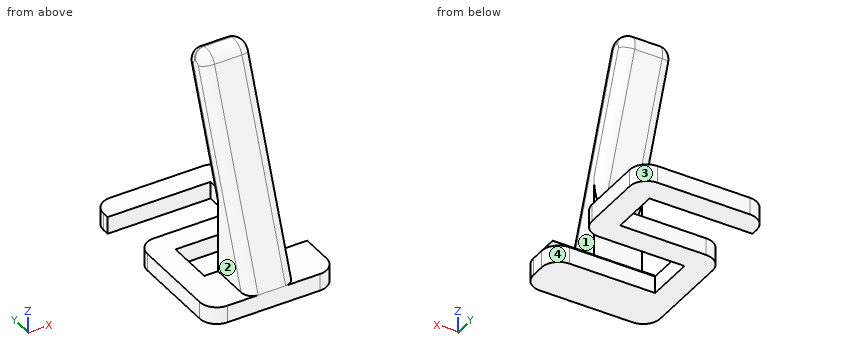
from build123d import *

# Parameters (mm, degrees)
F1_DEPTH = 5
F3_DEPTH = 37
F5_DEPTH = 36.2749
F6_R     = 4
F7_R     = 3
F8_R     = 4.99999


# Not quite as in the source:
# - a fillet or chamfer is up to 0.001 mm smaller than in the source, because OpenCascade refuses the exact size


with BuildPart() as f1:
    # F0 (on Top) → F1 (new body)
    with BuildSketch(Plane.XY):
        Polygon((0, 35), (0, 0), (37, 0), (37, 14), (7, 14), (7, 28), (37, 28), (37, 35), (37, 56), (0, 56), (0, 49), (30, 49), (30, 35), align=None)
    extrude(amount=F1_DEPTH)

    # F2 (on Right) → F3 (join)
    with BuildSketch(Plane.YZ):
        Polygon((22.2313093162, 66.0800203511), (0, 5), (9, 5), (14.2503125495, 4.9267373979), (14.2503125495, 19.4251151749), (30.1785093102, 63.1874761075), align=None)
    extrude(amount=F3_DEPTH)

    # F4 (on Front) → F5 (cut)
    with BuildSketch(Plane.XZ):
        Polygon((11, 5), (11, 66.0800203511), (25, 66.0800203511), (25, 5), (61.9937415394, 5), (61.9937415394, 77.6014764043), (-15.3317964795, 77.6014764043), (-15.3317964795, 5), align=None)
    extrude(amount=-F5_DEPTH, mode=Mode.SUBTRACT)

    # F6
    f6_edges = [f1.edges().sort_by_distance(p)[0] for p in [
        (18, 22.231309, 66.08002),
        (18, 30.178509, 63.187476),
    ]]
    fillet(f6_edges, radius=F6_R)

    # F7
    f7_edges = [f1.edges().sort_by_distance(p)[0] for p in [
        (11, 21.530371, 39.42691),
        (11, 10.431614, 33.660625),
        (25, 21.530371, 39.42691),
        (25, 10.431614, 33.660625),
    ]]
    fillet(f7_edges, radius=F7_R)

    # F8 (radius 5 in the source; OpenCascade refuses exactly that, so slightly less here)
    f8_edges = [f1.edges().sort_by_distance(p)[0] for p in [
        (37, 0, 2.5),
        (37, 28, 2.5),
        (37, 14, 2.465115),
        (0, 0, 2.5),
        (0, 35, 2.5),
        (0, 56, 2.5),
        (37, 56, 2.5),
    ]]
    fillet(f8_edges, radius=F8_R)


solid = f1.part
Design review of the part built by this model. Coordinates are the model's own, in mm. Face numbers are marked on the shaded views. A direction names the side the tool comes from. Coordinates: 2 decimals unless noted, no trailing zeros. Loops run counter-clockwise (first coordinate to the right, second up) from the corner with the lowest first, then second, coordinate; pieces in that order, holes last. Notation, with made-up numbers: (88.25, 15) -> (113.25, 15) arc R14 cw to (113.25, 40) -> close; hole circle Ø9 at (-9.5, 46.25). An arc over 180 degrees is marked (long way). Use a Markdown table: item, result. Add a question column.
Item 1: Wall thickness on L1, parallel to Z at x = 19.5, y = 53; L2, parallel to X at y = 13.5, z = 27; L3, parallel to Y at x = 12, z = 44.5: over which ranges is each line inside the solid? List them lowest first. Write a range as from..to.
Item 2: We need section C-C, the plane y = 42. Write out the cut boundary in (x, z), and give its area (3 significant figures).
Item 3: Machinability: for the marked faces 1, 2, 3 and 4, which of the approach directions +Z, -Z, +X, -X, +Y, -Y give a long, thin tool a straight path to every point of the face, cutting with its end or side? Answer none if there is none.
Item 4: Clearance check with flat-ended pins moving along their axes: P1, Ø1.5, axis at y = 22.5, z = 1.5, coming from the +X side; P2, Ø12, axis at x = 5.5, y = 47.5, coming from the +Z side; P3, Ø8, axis at x = 17.5, z = 38, coming from the -Y side; P4, Ø18.5, axis at x = 21.5, y = 31.5, coming from the +Z side. State where each tip first meets the part, or that it passes through.
Item 5: We need section A-A, the plane x = 10. Write out the cut boundary in (y, z).
Item 6: We need section B-B, the plane x = 18. Write out the cut boundary in (y, z).
Numbers:
| question | item | result |
|---|---|---|
| 1 | L1 | z = 0..5 |
| 1 | L2 | x = 11..25 |
| 1 | L3 | y = 15.19..22.56 |
| 2 | outline | (30, 0) -> (37, 0) -> (37, 5) -> (30, 5) -> close |
| 2 | area | 35.0 mm^2 |
| 3 | face 1 | +Z, +X, +Y, -Y |
| 3 | face 2 | +Z, -X, +Y, -Y |
| 3 | face 3 | +Z, -Z, +X, +Y |
| 3 | face 4 | -Z, +X |
| 4 | P1 | stops at x = 7 |
| 4 | P2 | stops at z = 5 |
| 4 | P3 | stops at y = 10.56 |
| 4 | P4 | stops at z = 64.95 |
| 5 | outline | (0, 0) -> (14, 0) -> (14, 4.93) -> (14.25, 4.93) -> (14.25, 5) -> (0, 5) -> close; (28, 0) -> (35, 0) -> (35, 5) -> (28, 5) -> close; (49, 0) -> (56, 0) -> (56, 5) -> (49, 5) -> close |
| 6 | outline | (0, 0) -> (14, 0) -> (14, 4.93) -> (14.25, 4.93) -> (14.25, 19.43) -> (28.81, 59.43) arc R4 ccw to (26.42, 64.56) -> (25.99, 64.71) arc R4 ccw to (20.86, 62.32) -> (0, 5) -> close; (28, 0) -> (35, 0) -> (35, 5) -> (28, 5) -> close; (49, 0) -> (56, 0) -> (56, 5) -> (49, 5) -> close |
